CAD build for the part. Positions are in the model's coordinates, mm. Face numbers are marked on the shaded views. A direction names the side the tool comes from. Coordinates: 2 decimals unless noted, no trailing zeros. Order: outer loops, then holes, each group sorted by start corner. A loop starts at its lowest first (then second) coordinate and runs counter-clockwise, first axis right, second up. Notation, with made-up numbers: (16.25, -10) - (50.25, -10) arc R25 ccw to (50.25, 20) - close; hole circle Ø9 at (-28.5, -34). An arc over 180 degrees is marked (long way). Use one line per item in the form item = value.
```python
from build123d import *

# Parameters (mm, degrees)
EXTRUDE_1_DEPTH      = 3
SKETCH_2_W           = 20
SKETCH_2_H           = 3
EXTRUDE_2_DEPTH      = 18
EXTRUDE_2_DEPTH_BACK = 3
SKETCH_5_R           = 1.6
CUT_EXTRUDE_1_DEPTH  = 31.938884609
CUT_EXTRUDE_2_DEPTH  = 4
EXTRUDE_3_DEPTH      = 3


with BuildPart() as part:
    # 草图1 → 凸台-拉伸1 (new body)
    with BuildSketch(Plane.XY):
        Polygon((-7.634327041, -2.906141593), (-7.634327041, 8.093858407), (12.365672959, 21.427191741), (12.365672959, -5.906141593), (-7.634327041, -5.906141593), align=None)
    extrude(amount=EXTRUDE_1_DEPTH)

    # 草图2 → 凸台-拉伸2 (add, two sides)
    with BuildSketch(Plane.XY.offset(3)) as extrude_2_sk:
        Polygon((-7.634327041, 8.093858407), (12.365672959, 21.427191741), (12.365672959, 25.032743016), (-7.634327041, 11.699409683), align=None)
        with Locations((2.365672959, -4.406141593)):
            Rectangle(SKETCH_2_W, SKETCH_2_H)
    extrude(amount=EXTRUDE_2_DEPTH)
    extrude(extrude_2_sk.sketch, amount=-EXTRUDE_2_DEPTH_BACK)

    # 草图5 → 切除-拉伸1 (cut, through all)
    with BuildSketch(Plane.XZ.offset(5.906141593)):
        with Locations((2.365672959, 8)):
            Circle(SKETCH_5_R)
    extrude(amount=-CUT_EXTRUDE_1_DEPTH, mode=Mode.SUBTRACT)

    # 草图6 → 切除-拉伸2 (cut, through all)
    with BuildSketch(Plane.XY.offset(3)):
        Polygon((-7.634327041, 8.093858407), (-7.634327041, -2.906141593), (12.365672959, -2.906141593), (12.365672959, 21.427191741), align=None)
    extrude(amount=-CUT_EXTRUDE_2_DEPTH, mode=Mode.SUBTRACT)

    # 草图7 → 凸台-拉伸3 (add)
    with BuildSketch(Plane.XY.offset(21)):
        Polygon((-7.634327041, 11.699409683), (-7.634327041, -5.906141593), (12.365672959, -5.906141593), (12.365672959, 25.032743016), align=None)
    extrude(amount=-EXTRUDE_3_DEPTH)


solid = part.part
```
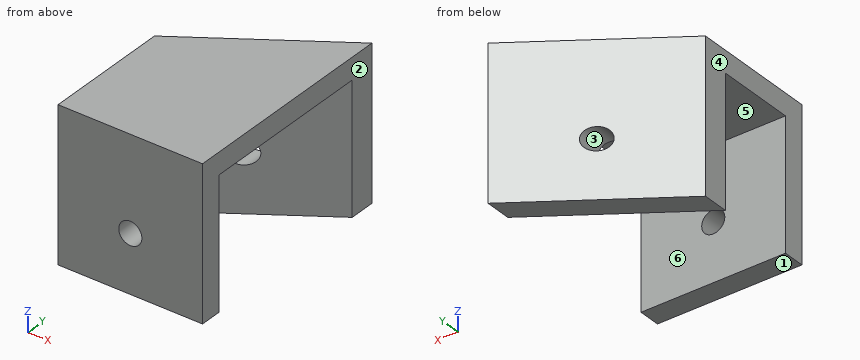
Item 1: Drop flat-ended pins along their axis: pin 1 (8 mm diameter, centred on x = -4.5, z = 18, fed in from +Y); pin 2 (9 mm diameter, centred on x = 4, z = 13, fed in from +Y); pin 3 (6 mm diameter, centred on x = 3.5, y = 19, fed in from -Z); pin 4 (2 mm diameter, centred on y = 8, z = 11.5, fed in from +X). Give the stop position or say it passes through.
Derived:
pin_1 = 16.46
pin_2 = 22.46
pin_3 = 0
pin_4 = -6.28
Item 2: Cut at B-B, the plane z = 8.75. Write the cut outline in (x, y), plus the area to 3 significant figures.
Derived:
outline = (-7.63, -5.91) - (0.95, -5.91) - (0.95, -2.91) - (-7.63, -2.91) - close; (-7.63, 8.09) - (0.95, 13.82) - (0.95, 17.42) - (-7.63, 11.7) - close; (3.78, -5.91) - (12.37, -5.91) - (12.37, -2.91) - (3.78, -2.91) - close; (3.78, 15.7) - (12.37, 21.43) - (12.37, 25.03) - (3.78, 19.31) - close
area = 113 mm²
Item 3: 3-axis set-ups, long thin cutter, end or side, ignore diameter. For the marked faces 4, 5 and 6: which of +Z, -Z, +X, -X, +Y, -Y reach the whole face in a straight line?
Derived:
face_4 = +Z, -Z, -X, +Y, -Y
face_5 = -Z, +X
face_6 = -Z, +X, -X
Item 4: Cut at D-D, the plane y = 13. Write the cut outline in (x, z), plus the area to 3 significant figures.
Derived:
outline = (-5.68, 0) - (-0.28, 0) - (-0.28, 18) - (12.37, 18) - (12.37, 21) - (-5.68, 21) - close
area = 151 mm²
Item 5: Cut at C-C, the plane x = -5.25. Write the cut outline in (y, z), plus the area to 3 significant figures.
Derived:
outline = (-5.91, 0) - (-2.91, 0) - (-2.91, 18) - (9.68, 18) - (9.68, 0) - (13.29, 0) - (13.29, 21) - (-5.91, 21) - close
area = 176 mm²
Item 6: Two-plate mould, pull along Z, no slides. Class the marked faces 1, 2 and 3: +Z half, -Z half, draft (parallel to the pull), parting line (faces both ways), or undercut.
Derived:
face_1 = -Z half
face_2 = draft
face_3 = undercut
Item 7: Drill centre lines: line 1 (Y direction, x = -6.25, z = 8.25); line 2 (Z direction, x = 1.5, y = 6); line 3 (Y direction, x = 0.25, z = 4.25). Where is each one in solid material? Low to high. Write a range as [from, to].
Derived:
line_1 = [-5.91, -2.91], [9.02, 12.62]
line_2 = [18, 21]
line_3 = [-5.91, -2.91], [13.35, 16.96]
Item 8: Cut at A-A, the plane z = 14. Write the cut outline in (x, y).
Derived:
outline = (-7.63, -5.91) - (12.37, -5.91) - (12.37, -2.91) - (-7.63, -2.91) - close; (-7.63, 8.09) - (12.37, 21.43) - (12.37, 25.03) - (-7.63, 11.7) - close
